```python
from build123d import *

# Parameters (mm, degrees)
F1_DEPTH = 25
F2_T     = -1.2
F3_R     = 20
F4_R     = 5


with BuildPart() as f1:
    # F0 (on Right) → F1 (new body, symmetric)
    with BuildSketch(Plane.YZ):
        Polygon((30, -10), (30, 20), (-30, 20), (-30, -20), (30, -20), align=None)
        Polygon((42, -10), (30, -10), (30, -20), align=None)
    extrude(amount=F1_DEPTH, both=True)

    # F2
    f2_openings = [f1.faces().sort_by_distance(p)[0] for p in [
        (0, 30, 5),
        (0, 36, -10),
    ]]
    offset(amount=F2_T, openings=f2_openings)

    # F3
    f3_edges = [f1.edges().sort_by_distance(p)[0] for p in [
        (0, 29.56554, -18.8),
    ]]
    fillet(f3_edges, radius=F3_R)

    # F4
    f4_edges = [f1.edges().sort_by_distance(p)[0] for p in [
        (-24.4, 30, -10),
        (24.4, 30, -10),
    ]]
    fillet(f4_edges, radius=F4_R)


solid = f1.part
```
The listing builds one solid part. Answer for the finished solid, in the listing's coordinates (mm). A direction names the side the tool comes from. Coordinates: 2 decimals unless noted, no trailing zeros. Loops run counter-clockwise (first coordinate to the right, second up) from the corner with the lowest first, then second, coordinate; pieces in that order, holes last. Notation, with made-up numbers: (48.25, 46.5) -> (63.25, 46.5) arc R8 ccw to (63.25, 54.5) -> close; hole circle Ø11 at (-23.75, -0.5). An arc over 180 degrees is marked (long way). Use one line per item in the form item = value. Start each with the question number.
Item 1: The part is cut by section B-B on z = 0. Determine the outline of the cut face in (x, y).
Item 2: The part is cut by section C-C on x = -10.5. Determine the outline of the cut face in (y, z).
Item 3: The part is cut by section A-A on y = -1.5. Determine the outline of the cut face in (x, z), then the cut area to 3 significant figures.
Item 4: A tool of negligible diameter and unlimited length cuts with its end or side. For faces 1 (the face through (0, 1, 18.8)), 2 (the face through (0, -30, 0)), 3 (the face through (23.8, 5, 0)), 4 (the face through (0.333, 37.592, -12.111)), 5 (the face through (0, 30, 19)), from which of +Z, -Z, +X, -X, +Y, -Y can it reach the whole face along a straight path? Write none if from no direction.
Item 5: Flat-ended cylindrical pins translate along their axes: pin 1 Ø2 at (x, z) = (4.5, 14) entering from +Y; pin 2 Ø7.5 at (x, y) = (0, 37) entering from +Z. Find the tip coordinate at first contact, or state that the pin passes through.
Item 6: The mould has two halves that part along X. Classify faces 6 (the face through (-24, 32, -9)), 7 (the face through (-25, 5, 0)), 8 (the face through (0, -4, -18.8)), 9 (the face through (0, -28.8, 0)): released by +X, released by -X, zero draft, split by the parting line, or undercut.
Item 7: Consider L1, parallel to X at y = 24, z = -4; L2, parallel to Z at x = 20, y = 4; L3, parallel to Y at x = -0.5, z = -4.5. Determine where each line is inside the solid, lowest interval first. Write a range as [from, to].
Item 8: The part is cut by section D-D on z = -16. Determine the outline of the cut face in (x, y).
Answer key:
q1.outline = (-25, -30) -> (25, -30) -> (25, 30) -> (23.8, 30) -> (23.8, -28.8) -> (-23.8, -28.8) -> (-23.8, 30) -> (-25, 30) -> close
q2.outline = (-30, -20) -> (30, -20) -> (42, -10) -> (40.13, -10) -> (35.13, -14.16) arc R20 cw to (22.32, -18.8) -> (-28.8, -18.8) -> (-28.8, 18.8) -> (30, 18.8) -> (30, 20) -> (-30, 20) -> close
q3.outline = (-25, -20) -> (25, -20) -> (25, 20) -> (-25, 20) -> close; hole (-23.8, -18.8) -> (23.8, -18.8) -> (23.8, 18.8) -> (-23.8, 18.8) -> close
q3.area = 210 mm2
q4.face_1 = +Y
q4.face_2 = +Z, -Z, +X, -X, -Y
q4.face_3 = none
q4.face_4 = +Z
q4.face_5 = +Z, +X, -X, +Y
q5.pin_1 = -28.8
q5.pin_2 = -10
q6.face_6 = zero draft
q6.face_7 = released by -X
q6.face_8 = undercut
q6.face_9 = undercut
q7.L1 = [-25, -23.8], [23.8, 25]
q7.L2 = [-20, -18.8], [18.8, 20]
q7.L3 = [-30, -28.8]
q8.outline = (-25, -30) -> (25, -30) -> (25, 34.8) -> (-25, 34.8) -> close; hole (-23.8, -28.8) -> (23.8, -28.8) -> (23.8, 32.53) -> (-23.8, 32.53) -> close
